from build123d import *

# Parameters (mm, degrees)
FILLET1_R      = 0.1
FILLET2_R      = 0.12
CHAMFER1_SIZE  = 0.2
EXTRUDE1_DEPTH = 1


with BuildPart() as part:
    # Sketch1 → Revolve1 (revolve)
    with BuildSketch(Plane.XY, mode=Mode.PRIVATE) as revolve1_sk:
        Polygon((2, 1.5), (2, 0), (4.279914881, 0), (14, 0), (14, 1.5), align=None)
        Polygon((0, 2.75), (0, 0), (2, 0), (2, 1.5), (2, 2.75), align=None)
    revolve(revolve1_sk.sketch.rotate(Axis((0, 0, 0), (1, 0, 0)), 90), axis=Axis((0, 0, 0), (1, 0, 0)))

    # Fillet1
    fillet1_edges = [part.edges().sort_by_distance(p)[0] for p in [
        (2, 0, -1.5),
    ]]
    fillet(fillet1_edges, radius=FILLET1_R)

    # Fillet2
    fillet2_edges = [part.edges().sort_by_distance(p)[0] for p in [
        (0, 0, -2.75),
    ]]
    fillet(fillet2_edges, radius=FILLET2_R)

    # Chamfer1
    chamfer1_edges = [part.edges().sort_by_distance(p)[0] for p in [
        (14, 0, -1.5),
    ]]
    chamfer(chamfer1_edges, length=CHAMFER1_SIZE)

    # Sketch2 → Extrude1 (cut)
    with BuildSketch(Plane.ZY):
        Polygon((0, 1.443375673), (-1.25, 0.721687836), (-1.25, -0.721687836), (0, -1.443375673), (1.25, -0.721687836), (1.25, 0.721687836), align=None)
    extrude(amount=-EXTRUDE1_DEPTH, mode=Mode.SUBTRACT)


solid = part.part
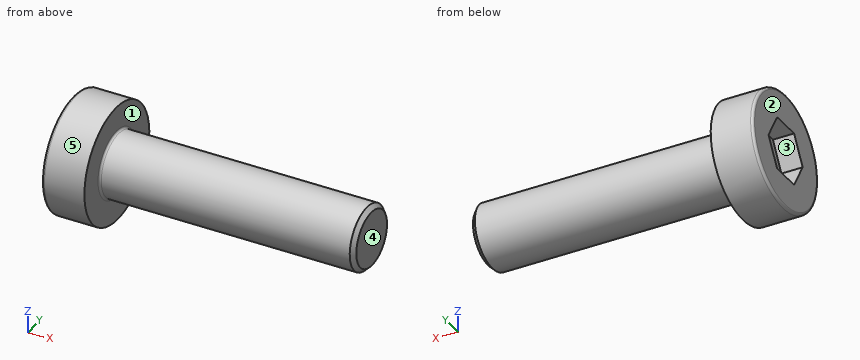
Can you work these out from the model? Positions are in its coordinate system, mm. Face numbers are marked on the shaded views. A direction names the side the tool comes from. Round coordinates to 2 decimals unless told otherwise and drop trailing zeros. Loops run counter-clockwise (first coordinate to the right, second up) from the corner with the lowest first, then second, coordinate; pieces in that order, holes last. Notation, with made-up numbers: (21.25, -25.75) - (45.25, -25.75) arc R24 cw to (45.25, -3.75) - close; hole circle Ø1 at (-39.5, -17.5). An arc over 180 degrees is marked (long way). Write item = value, one per line. Start each with the question number.
(1) If we section it at B-B (x = 6.5): Please give me the cut outline in (y, z), and give its area (3 significant figures).
(2) For P1, Ø3, axis at x = 8, y = -2, coming from the +Z side; P2, Ø3, axis at x = 2.5, z = 0.5, coming from the +Y side; P3, Ø0.8, axis at y = 0, z = 0, coming from the -X side, each with a flat end and sliding along its axis, tell me the tip position at first contact or that it passes through.
(3) If I drill on probe 1 along Y at (x, z) = (3.5, -0.1); probe 2 along X at (y, z) = (0.9, -1.8); probe 3 along X at (y, z) = (0.65, -0.1), over which ranges is the centre line in solid material (lowest first)? Write a range as [from, to].
(4) If we mould it in two halves opening along Z, with no side actions, what happens to the marked faces 3, 4 and 5? For each: released by +Z, released by -Z, zero draft, split by the parting line, or undercut.
(5) For the marked faces 1 and 2, which set-ups out of +Z, -Z, +X, -X, +Y, -Y let a thin tool reach every point of the face, with its end or its side?
(6) If we section it at A-A (y = 0): Please give me the cut outline in (x, z).
Ans:
q1.outline = circle Ø3 at (0, 0)
q1.area = 7.07 mm²
q2.P1 = 1.41
q2.P2 = 2.75
q2.P3 = 1
q3.probe_1 = [-1.5, 1.5]
q3.probe_2 = [0, 2]
q3.probe_3 = [1, 14]
q4.face_3 = undercut
q4.face_4 = zero draft
q4.face_5 = split by the parting line
q5.face_1 = +X
q5.face_2 = +Z, -Z, -X, +Y, -Y
q6.outline = (0, -2.63) arc R0.12 ccw to (0.12, -2.75) - (2, -2.75) - (2, -1.6) arc R0.1 cw to (2.1, -1.5) - (13.8, -1.5) - (14, -1.3) - (14, 1.3) - (13.8, 1.5) - (2.1, 1.5) arc R0.1 cw to (2, 1.6) - (2, 2.75) - (0.12, 2.75) arc R0.12 ccw to (0, 2.63) - (0, 1.25) - (1, 1.25) - (1, -1.25) - (0, -1.25) - close
